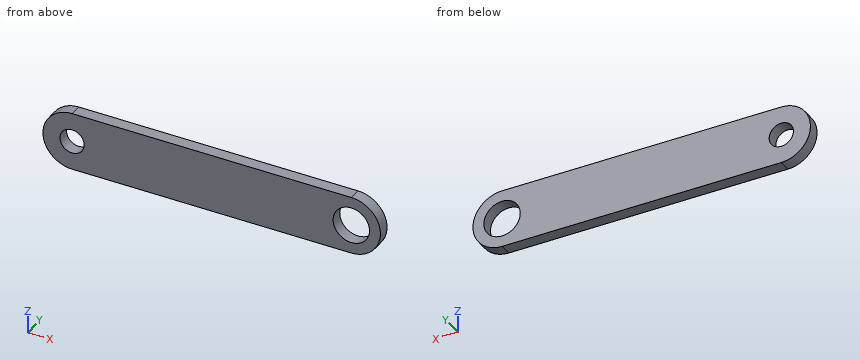
```python
from build123d import *

# Parameters (mm, degrees)
SKETCH1_R           = 5
SKETCH1_R_2         = 7.5
BOSS_EXTRUDE1_DEPTH = 5
SCALE2_SCALE        = 0.2004


with BuildPart() as part:
    # Sketch1 → Boss-Extrude1 (new body)
    with BuildSketch(Plane(origin=(0, 0, 0), x_dir=(1, 0, 0), z_dir=(0, 1, 0))):
        with BuildLine():
            Line((-57.5, 12), (57.5, 12))
            ThreePointArc((57.5, 12), (69.5, 0), (57.5, -12))
            Line((57.5, -12), (-57.5, -12))
            ThreePointArc((-57.5, -12), (-69.5, 0), (-57.5, 12))
        make_face()
        with Locations(Location((-57.5, 0, 0), (0, 0, 270))):
            Circle(SKETCH1_R, mode=Mode.SUBTRACT)
        with Locations(Location((57.5, 0, 0), (0, 0, 270))):
            Circle(SKETCH1_R_2, mode=Mode.SUBTRACT)
    extrude(amount=BOSS_EXTRUDE1_DEPTH)


with BuildPart() as part_1:
    # Scale2: scaled about (-1.908958981, 2.5, 0)
    add(part.part.scale(SCALE2_SCALE).moved(Location((-1.526403601, 1.999, 0))))


solid = part_1.part
```
Design review of the part built by this model. Coordinates are the model's own, in mm. Coordinates: 2 decimals unless noted, no trailing zeros. Order: outer loops, then holes, each group sorted by start corner. A loop starts at its lowest first (then second) coordinate and runs counter-clockwise, first axis right, second up. Notation, with made-up numbers: (78, 15.25) - (118, 15.25) arc R4 ccw to (118, 19.25) - close; hole circle Ø4 at (57, 45). An arc over 180 degrees is marked (long way). Answer in a Markdown table with one row per item.
(1) Consider section A-A on z = 0. State the section outline as (x, y) points, plus the area to 3 significant figures.
Checked values:
| item | result |
|---|---|
| outline | (-15.45, 2) - (-14.05, 2) - (-14.05, 3) - (-15.45, 3) - close; (-12.05, 2) - (8.49, 2) - (8.49, 3) - (-12.05, 3) - close; (11.5, 2) - (12.4, 2) - (12.4, 3) - (11.5, 3) - close |
| area | 22.9 mm^2 |
(2) Consider section B-B on y = 2.6. State the section outline as (x, z) points.
Checked values:
| item | result |
|---|---|
| outline | (-13.05, -2.4) - (10, -2.4) arc R2.4 ccw to (10, 2.4) - (-13.05, 2.4) arc R2.4 ccw to start; hole circle Ø2 at (-13.05, 0); hole circle Ø3.01 at (10, 0) |
(3) Wall thickness on line 1 along X through (y, z) = (2.4, 0); line 2 along X through (y, z) = (2.9, -1.2); line 3 along X through (y, z) = (2.1, 1.25): over which ranges is each line inside the solid? List them lowest first. Write a range as from..to.
Checked values:
| item | result |
|---|---|
| line 1 | -15.45..-14.05, -12.05..8.49, 11.5..12.4 |
| line 2 | -15.13..9.09, 10.9..12.08 |
| line 3 | -15.1..9.16, 10.83..12.05 |
(4) Consider section C-C on z = -2. State the section outline as (x, y) points.
Checked values:
| item | result |
|---|---|
| outline | (-14.38, 2) - (11.33, 2) - (11.33, 3) - (-14.38, 3) - close |
